```python
from build123d import *

# Parameters (mm, degrees)
SKETCH_1_R      = 5
EXTRUDE_1_DEPTH = 1
SKETCH_2_R      = 0.622519756
EXTRUDE_2_DEPTH = 80
SKETCH_3_W      = 4.001607156
SKETCH_3_H      = 1.375795034
EXTRUDE_3_DEPTH = 0.05


with BuildPart() as part:
    # 草图1 → 凸台-拉伸1 (new body)
    with BuildSketch(Plane(origin=(0, 0, 0), x_dir=(1, 0, 0), z_dir=(0, 1, 0))):
        with Locations(Location((0, 0, 0), (0, 0, 270))):
            Circle(SKETCH_1_R)
    extrude(amount=EXTRUDE_1_DEPTH)

    # 草图2 → 凸台-拉伸2 (add)
    with BuildSketch(Plane(origin=(0, 0, 0), x_dir=(1, 0, 0), z_dir=(0, 1, 0))):
        with Locations(Location((0, 0, 0), (0, 0, 270))):
            Circle(SKETCH_2_R)
    extrude(amount=EXTRUDE_2_DEPTH)

    # 草图3 → 凸台-拉伸3 (add, symmetric)
    with BuildSketch(Plane.XY):
        with Locations((0.019961676, 0.687897517)):
            Rectangle(SKETCH_3_W, SKETCH_3_H)
    extrude(amount=EXTRUDE_3_DEPTH, both=True)


solid = part.part
```
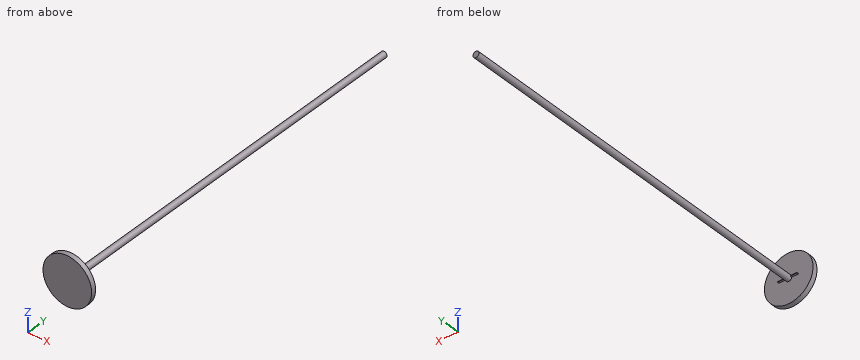
Design review of the part built by this model. Coordinates are the model's own, in mm. Coordinates: 2 decimals unless noted, no trailing zeros. Loops run counter-clockwise (first coordinate to the right, second up) from the corner with the lowest first, then second, coordinate; pieces in that order, holes last.
Q1. To check wall thickness, follow line 1 (Y direction, x = 2.5, z = 2.5); line 2 (Y direction, x = -1.25, z = 0); line 3 (X direction, y = 62, z = 0). State the ranges of each line that lie inside material, in increasing order.
Reported:
line 1: y = 0 to 1
line 2: y = 0 to 1.38
line 3: x = -0.62 to 0.62
Q2. We need section A-A on x = -3. State the section outline as (y, z) points, and give its area (3 significant figures).
Reported:
outline: (0, -4) - (1, -4) - (1, 4) - (0, 4) - close
area: 8.00 mm2
Q3. We need section B-B on y = 36. State the section outline as (x, z) points.
Reported:
outline: circle Ø1.25 at (0, 0)
Q4. For pin 1 (1 mm diameter, centred on x = -2.5, y = 53, fed in from +Z); pin 2 (1.5 mm diameter, centred on x = -0.5, z = 2.5, fed in from +Y); pin 3 (1 mm diameter, centred on y = 41, z = 0.5, fed in from -X), all flat-tipped, find the tip position at first contact; note any pin that passes through.
Reported:
pin 1: passes through
pin 2: stops at y = 1
pin 3: stops at x = -0.62
Q5. We need section C-C on z = 4. State the section outline as (x, y) points, and give its area (3 significant figures).
Reported:
outline: (-3, 0) - (3, 0) - (3, 1) - (-3, 1) - close
area: 6.00 mm2
